from build123d import *

# Parameters (mm, degrees)
SKETCH_1_R      = 10
SKETCH_1_R_2    = 1.5
EXTRUDE_1_DEPTH = 2
SKETCH_2_R      = 4.5
SKETCH_2_R_2    = 3
EXTRUDE_2_DEPTH = 2


with BuildPart() as part:
    # 草图1 → 凸台-拉伸1 (new body)
    with BuildSketch(Plane.XY):
        Circle(SKETCH_1_R)
        Circle(SKETCH_1_R_2, mode=Mode.SUBTRACT)
        with Locations((0, 7)):
            Circle(SKETCH_1_R_2, mode=Mode.SUBTRACT)
        with Locations((7, 0)):
            Circle(SKETCH_1_R_2, mode=Mode.SUBTRACT)
        with Locations((0, -7)):
            Circle(SKETCH_1_R_2, mode=Mode.SUBTRACT)
        with Locations((-7, 0)):
            Circle(SKETCH_1_R_2, mode=Mode.SUBTRACT)
    extrude(amount=EXTRUDE_1_DEPTH)

    # 草图2 → 凸台-拉伸2 (add)
    with BuildSketch(Plane(origin=(0, 0, 0), x_dir=(-1, 0, 0), z_dir=(0, 0, -1))):
        with Locations(Location((0, 0, 0), (0, 0, 180))):
            Circle(SKETCH_2_R)
        Circle(SKETCH_2_R_2, mode=Mode.SUBTRACT)
    extrude(amount=EXTRUDE_2_DEPTH)


solid = part.part
Geometry: final body of the model. Coordinates: model frame, mm. A direction names the side the tool comes from. Give positions to 0.01 mm unless a question says otherwise; leave off trailing zeros. Loops run counter-clockwise (first coordinate to the right, second up) from the corner with the lowest first, then second, coordinate; pieces in that order, holes last. Notation, with made-up numbers: (-6, 52) -> (23, 52) arc R10 cw to (23, 59) -> close; hole circle Ø6 at (49.5, 48). An arc over 180 degrees is marked (long way). Put each result on its own line as item: value.
1. Ray query, line 1 along Y through (x, z) = (0, 0.55); line 2 along Z through (x, y) = (-1.5, -8.25); line 3 along X through (y, z) = (-1.25, 0.75). Return the intervals inside material, ascending. Write a range as [from, to].
Taken from the geometry:
line 1: y = [-10, -8.5], [-5.5, -1.5], [1.5, 5.5], [8.5, 10]
line 2: z = [0, 2]
line 3: x = [-9.92, -7.83], [-6.17, -0.83], [0.83, 6.17], [7.83, 9.92]
2. Set-up query: faces 4 (the flat face through (1.3, -1.3, 0)), 5 (the cylindrical face through (-2.17, -9.76, 0.99)). Return all of +Z, -Z, +X, -X, +Y, -Y with unobstructed straight access to the full face (end or side cutting, diameter ignored); none if empty.
Taken from the geometry:
face 4: -Z
face 5: +Z, -Z
3. Cut plane C-C (y = 5.75). Return the cut outline in (x, z).
Taken from the geometry:
outline: (-8.18, 0) -> (-0.83, 0) -> (-0.83, 2) -> (-8.18, 2) -> close; (0.83, 0) -> (8.18, 0) -> (8.18, 2) -> (0.83, 2) -> close
4. Pull-direction query (Y, two-part tool) for faces 1 (the flat face through (1, 3, -2)), 2 (the cylindrical face through (-0.325, 5.536, 0.986)), 3 (the cylindrical face through (-3.32, -3.04, -0.99)); classes: released by +Y, released by -Y, zero draft, split by the parting line, or undercut.
Taken from the geometry:
face 1: zero draft
face 2: undercut
face 3: split by the parting line
5. Cut plane D-D (z = 0.75). Return the cut outline in (x, y), plus the area to 3 significant figures.
Taken from the geometry:
outline: circle Ø20 at (0, 0); hole circle Ø3 at (-7, 0); hole circle Ø3 at (0, -7); hole circle Ø3 at (0, 0); hole circle Ø3 at (0, 7); hole circle Ø3 at (7, 0)
area: 279 mm2
6. Cut plane A-A (x = 0). Return the cut outline in (y, z).
Taken from the geometry:
outline: (-10, 0) -> (-8.5, 0) -> (-8.5, 2) -> (-10, 2) -> close; (-5.5, 0) -> (-4.5, 0) -> (-4.5, -2) -> (-3, -2) -> (-3, 0) -> (-1.5, 0) -> (-1.5, 2) -> (-5.5, 2) -> close; (1.5, 0) -> (3, 0) -> (3, -2) -> (4.5, -2) -> (4.5, 0) -> (5.5, 0) -> (5.5, 2) -> (1.5, 2) -> close; (8.5, 0) -> (10, 0) -> (10, 2) -> (8.5, 2) -> close
7. Pin query (flat end, axial travel): P1, Ø1, axis at x = 4, z = -1.5, coming from the +Y side; P2, Ø1, axis at x = -1, z = 0, coming from the +Y side. Return the tip coordinate at first contact, or that it passes through.
Taken from the geometry:
P1: stops at y = 2.83
P2: stops at y = 9.99
